```python
from build123d import *

# Parameters (mm, degrees)
BOSS_EXTRUDE1_DEPTH                 = 6.35
FILLET1_R                           = 6.35
FILLET2_R                           = 2.54
FILLET3_R                           = 1.27
F_8_32_TAPPED_HOLE3_D               = 4
F_8_32_TAPPED_HOLE3_DEPTH           = 10.70864
F_8_32_TAPPED_HOLE3_TIP             = 1.201721238
F_8_32_TAPPED_HOLE3_ON_FACE_2_D     = 4
F_8_32_TAPPED_HOLE3_ON_FACE_2_DEPTH = 10.70864
F_8_32_TAPPED_HOLE3_ON_FACE_2_TIP   = 1.201721238
F_8_32_TAPPED_HOLE3_ON_FACE_3_D     = 4
F_8_32_TAPPED_HOLE3_ON_FACE_3_DEPTH = 10.70864
F_8_32_TAPPED_HOLE3_ON_FACE_3_TIP   = 1.201721238


with BuildPart() as part:
    # Sketch1 → Boss-Extrude1 (new body)
    with BuildSketch(Plane.XY):
        Polygon((-11.971057013, -34.21026192), (-5.816733064, -35.774485923), (-3.470397058, -26.543), (3.470397058, -26.543), (5.816733064, -35.774485923), (11.971057013, -34.21026192), (7.601357108, -17.018), (-7.601357108, -17.018), align=None)
    extrude(amount=BOSS_EXTRUDE1_DEPTH)

    # Fillet1
    fillet1_edges = [part.edges().sort_by_distance(p)[0] for p in [
        (-7.601357108, -17.018, 3.175),
        (7.601357108, -17.018, 3.175),
    ]]
    fillet(fillet1_edges, radius=FILLET1_R)

    # Fillet2
    fillet2_edges = [part.edges().sort_by_distance(p)[0] for p in [
        (3.470397058, -26.543, 3.175),
        (-3.470397058, -26.543, 3.175),
    ]]
    fillet(fillet2_edges, radius=FILLET2_R)

    # Fillet3
    fillet3_edges = [part.edges().sort_by_distance(p)[0] for p in [
        (-5.816733064, -35.774485923, 3.175),
        (-11.971057013, -34.21026192, 3.175),
        (11.971057013, -34.21026192, 3.175),
        (5.816733064, -35.774485923, 3.175),
    ]]
    fillet(fillet3_edges, radius=FILLET3_R)

    # #8-32 Tapped Hole3
    with Locations(Plane(origin=(-8.893895038, -34.992373921, 3.175), x_dir=(-0.969184873822, 0.246334488763, 0), z_dir=(-0.246334488763, -0.969184873822, 0))):
        with Locations((0, 0)):
            Hole(F_8_32_TAPPED_HOLE3_D / 2, depth=F_8_32_TAPPED_HOLE3_DEPTH)
            with Locations((0, 0, -(F_8_32_TAPPED_HOLE3_DEPTH + F_8_32_TAPPED_HOLE3_TIP / 2))):  # 118° drill point
                Cone(0, F_8_32_TAPPED_HOLE3_D / 2, F_8_32_TAPPED_HOLE3_TIP, mode=Mode.SUBTRACT)

    # #8-32 Tapped Hole3 on face 2
    with Locations(Plane(origin=(8.893895038, -34.992373921, 3.175), x_dir=(-0.969184998168, -0.246333999534, 0), z_dir=(0.246333999534, -0.969184998168, 0))):
        with Locations((0, 0)):
            Hole(F_8_32_TAPPED_HOLE3_ON_FACE_2_D / 2, depth=F_8_32_TAPPED_HOLE3_ON_FACE_2_DEPTH)
            with Locations((0, 0, -(F_8_32_TAPPED_HOLE3_ON_FACE_2_DEPTH + F_8_32_TAPPED_HOLE3_ON_FACE_2_TIP / 2))):  # 118° drill point
                Cone(0, F_8_32_TAPPED_HOLE3_ON_FACE_2_D / 2, F_8_32_TAPPED_HOLE3_ON_FACE_2_TIP, mode=Mode.SUBTRACT)

    # #8-32 Tapped Hole3 on face 3
    with Locations(Plane(origin=(0, -17.018, 3.175), x_dir=(0, 0, 1), z_dir=(0, 1, 0))):
        with Locations((0, 0)):
            Hole(F_8_32_TAPPED_HOLE3_ON_FACE_3_D / 2, depth=F_8_32_TAPPED_HOLE3_ON_FACE_3_DEPTH)
            with Locations((0, 0, -(F_8_32_TAPPED_HOLE3_ON_FACE_3_DEPTH + F_8_32_TAPPED_HOLE3_ON_FACE_3_TIP / 2))):  # 118° drill point
                Cone(0, F_8_32_TAPPED_HOLE3_ON_FACE_3_D / 2, F_8_32_TAPPED_HOLE3_ON_FACE_3_TIP, mode=Mode.SUBTRACT)


solid = part.part
```
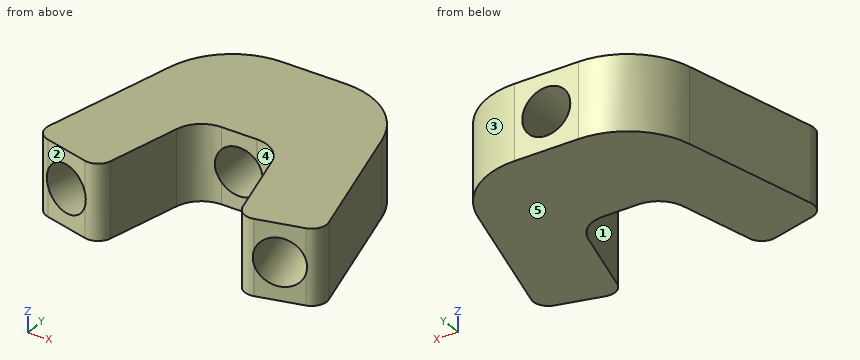
Work out the finished part from the listing and answer in its coordinate system (mm). Face numbers are marked on the shaded views. A direction names the side the tool comes from. Round coordinates to 2 decimals unless told otherwise and drop trailing zeros. Write each loop counter-clockwise with the first axis right and the second up, starting at its lowest first coordinate (ties: lowest second). Pieces come first, ordered by that corner, then holes.
1) A cutting plane is placed at B-B on z = 5.75. Determine the outline of the cut face in (x, y), and give its area (3 significant figures).
2) A cutting plane is placed at D-D on y = -20.75. Determine the outline of the cut face in (x, z) (3 decimals).
3) Determine the mould class of the marked faces 1, 2 and 3 for opening direction X: pulls with the +X half, pulls with the -X half, needs draft (parallel to the pull), parting line crosses it, or undercut.
4) Consider probe 1 along X at (y, z) = (-27.5, 4.5); probe 2 along X at (y, z) = (-27.25, 3); probe 3 along Z at (x, y) = (0, -19.5) (3 decimals). Determine where each line is inside the solid, lowest interval first.
5) Which of the six approach directions +Z, -Z, +X, -X, +Y, -Y give full straight-line access (tool end or side, diameter ignored) to the marked faces 4 and 5?
6) A cutting plane is placed at A-A on x = 0. Determine the outline of the cut face in (y, z) (3 decimals).
7) A cutting plane is placed at C-C on y = -34. Give the number of separate pieces and of enclosed holes in the cut face, and give its area (3 significant figures).
8) Flat-ended cylindrical pins translate along their axes: P1, Ø2, axis at y = -28.5, z = 4, coming from the -X side; P2, Ø0.9, axis at x = -0.5, z = 1, coming from the -Y side; P3, Ø2.5, axis at x = 0, z = 3.175, coming from the -Y side; P4, Ø2, axis at y = -24.5, z = 2.5, coming from the -X side. Find the tip coordinate at first contact, or state that the pin passes through.
Entries:
1. outline: (-11.66, -32.98) arc R1.27 ccw to (-10.74, -34.52) - (-7.05, -35.46) arc R1.27 ccw to (-5.5, -34.54) - (-3.96, -28.46) arc R2.54 cw to (-1.5, -26.54) - (1.5, -26.54) arc R2.54 cw to (3.96, -28.46) - (5.5, -34.54) arc R1.27 ccw to (7.05, -35.46) - (10.74, -34.52) arc R1.27 ccw to (11.66, -32.98) - (8.82, -21.8) arc R6.35 ccw to (2.66, -17.02) - (-2.66, -17.02) arc R6.35 ccw to (-8.82, -21.8) - close
1. area: 269 mm2
2. outline: (-8.449, 0) - (8.449, 0) - (8.449, 6.35) - (-8.449, 6.35) - close; hole circle Ø4 at (0, 3.175)
3. face 1: undercut
3. face 2: pulls with the -X half
3. face 3: pulls with the +X half
4. probe 1: x = -10.27 to -8.54, -5.44 to -3.48, 3.48 to 5.44, 8.54 to 10.27
4. probe 2: x = -10.2 to -8.98, -4.87 to -3.25, 3.25 to 4.87, 8.98 to 10.2
4. probe 3: z = 0 to 1.175, 5.175 to 6.35
5. face 4: +Z, -Z, -Y
5. face 5: -Z, +X, -X, +Y, -Y
6. outline: (-26.543, 0) - (-17.018, 0) - (-17.018, 1.175) - (-26.543, 1.175) - close; (-26.543, 5.175) - (-17.018, 5.175) - (-17.018, 6.35) - (-26.543, 6.35) - close
7. separate pieces: 2
7. enclosed holes: 2
7. area: 51.7 mm2
8. P1: stops at x = -10.77
8. P2: stops at y = -26.54
8. P3: passes through
8. P4: stops at x = -9.76
